Part model, mm, in its own coordinate system. Face numbers are marked on the shaded views. Coordinates: 2 decimals unless noted, no trailing zeros. Loops run counter-clockwise (first coordinate to the right, second up) from the corner with the lowest first, then second, coordinate; pieces in that order, holes last. Notation, with made-up numbers: (18, -25.75) - (71, -25.75) arc R29 ccw to (71, -2.75) - close; hole circle Ø7 at (28.5, 76.5). An arc over 180 degrees is marked (long way). Use a Markdown table: item, result. Add a question column.
1. Wall check: probe 1 along X at (y, z) = (99.5, 0); probe 2 along X at (y, z) = (-85.5, -11); probe 3 along Z at (x, y) = (-12, 92.5). Give the ranges that are in metal, low to high. Write a range as [from, to].
2. Drop flat-ended pins along their axis: pin 1 (5 mm diameter, centred on y = 34.5, z = 10, fed in from +X); pin 2 (2 mm diameter, centred on x = -2, z = -8.5, fed in from -Y); pin 3 (1 mm diameter, centred on x = 12.5, y = 90, fed in from +Z); pin 4 (4 mm diameter, centred on y = -31, z = -18.5, fed in from +X). Give the stop position or say it passes through.
3. Band-saw the part on A-A, the plane x = -10. Give the cut face in (y, z).
4. Pull direction Y, two halves, no side cores. Call the marked faces 1, 2, 3 and 4: pulls with the +Y half, pulls with the -Y half, needs draft (parallel to the pull), parting line crosses it, or undercut.
5. Band-saw the part on C-C, the plane x = 15. Give the cut face in (y, z), plus the area to 3 significant figures.
6. Band-saw the part on B-B, the plane z = 0. Give the cut face in (x, y).
from build123d import *

# Parameters (mm, degrees)
BOSS_EXTRUDE1_DEPTH = 7.5
CHAMFER1_SIZE       = 2.5
SKETCH2_R           = 5
BOSS_EXTRUDE2_DEPTH = 10
BOSS_EXTRUDE3_DEPTH = 5


with BuildPart() as part:
    # Sketch1 → Boss-Extrude1 (new, symmetric)
    with BuildSketch(Plane.YZ):
        with BuildLine():
            ThreePointArc((-81.871756055, 19.753837344), (-104.803696773, 2.795280684), (-87.461525308, -19.847944306))
            ThreePointArc((-87.461525308, -19.847944306), (0.380210023, -22.09713345), (86.984359422, -7.232725467))
            ThreePointArc((86.984359422, -7.232725467), (92.427584063, 1.039709088), (84.922137279, 7.499595816))
            ThreePointArc((84.922137279, 7.499595816), (1.268561005, 10.133701432), (-81.871756055, 19.753837344))
        make_face()
    extrude(amount=BOSS_EXTRUDE1_DEPTH, both=True)

    # Chamfer1
    chamfer1_edges = [part.edges().sort_by_distance(p)[0] for p in [
        (-7.5, 0.380210023, -22.09713345),
        (-7.5, -104.803696773, 2.795280684),
        (-7.5, 1.268561005, 10.133701432),
        (7.5, 0.380210023, -22.09713345),
        (7.5, -104.803696773, 2.795280684),
        (7.5, 1.268561005, 10.133701432),
    ]]
    chamfer(chamfer1_edges, length=CHAMFER1_SIZE)

    # Sketch2 → Boss-Extrude2 (add)
    with BuildSketch(Plane(origin=(-7.5, 0, 0), x_dir=(0, -1, 0), z_dir=(-1, 0, 0))):
        with Locations(Location((85, 0, 0), (0, 0, 270))):
            Circle(SKETCH2_R)
    extrude(amount=BOSS_EXTRUDE2_DEPTH)

    # Sketch4 → Boss-Extrude3 (add, symmetric)
    with BuildSketch(Plane(origin=(0, 0, 0), x_dir=(0, 1, 0), z_dir=(0, 0, 1))):
        with BuildLine():
            ThreePointArc((86.984359422, 0), (95.845428844, -15.310516356), (113.386137378, -17.602678336))
            ThreePointArc((113.386137378, -17.602678336), (115.102678336, -14.113862622), (111.613862622, -12.397321664))
            ThreePointArc((111.613862622, -12.397321664), (99.049040037, -10.836148037), (92.5, 0))
            ThreePointArc((92.5, 0), (99.049040037, 10.836148037), (111.613862622, 12.397321664))
            ThreePointArc((111.613862622, 12.397321664), (115.102678336, 14.113862622), (113.386137378, 17.602678336))
            ThreePointArc((113.386137378, 17.602678336), (95.845428844, 15.310516356), (86.984359422, 0))
        make_face()
    extrude(amount=BOSS_EXTRUDE3_DEPTH, both=True)


solid = part.part
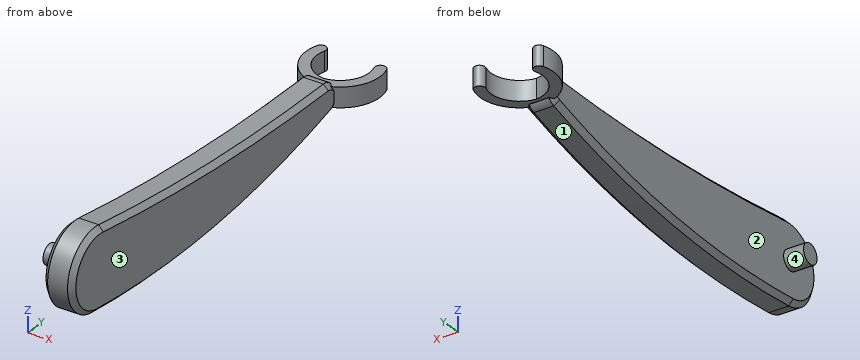
Geometry check:
| question | item | result |
|---|---|---|
| 1 | probe 1 | x = [-17.23, -11.12], [11.12, 17.23] |
| 1 | probe 2 | x = [-7.5, 7.5] |
| 1 | probe 3 | z = [-5, 5] |
| 2 | pin 1 | stops at x = 5.75 |
| 2 | pin 2 | stops at y = -103.54 |
| 2 | pin 3 | passes through |
| 2 | pin 4 | stops at x = 7.5 |
| 3 | outline | circle Ø10 at (-85, 0); (90.46, -5) - (97.89, -5) - (97.89, 5) - (90.46, 5) - close |
| 4 | face 1 | parting line crosses it |
| 4 | face 2 | undercut |
| 4 | face 3 | needs draft |
| 4 | face 4 | undercut |
| 5 | outline | (95.39, -5) - (115.25, -5) - (115.25, 5) - (95.39, 5) - close |
| 5 | area | 199 mm^2 |
| 6 | outline | (-17.6, 113.39) arc R20 ccw to (-7.5, 88.99) - (-7.5, -80) - (-17.5, -80) - (-17.5, -90) - (-7.5, -90) - (-7.5, -102.5) - (-5, -105) - (5, -105) - (7.5, -102.5) - (7.5, 88.99) arc R20 ccw to (17.6, 113.39) arc R2.75 ccw to (12.4, 111.61) arc R14.5 cw to (0, 92.5) arc R14.5 cw to (-12.4, 111.61) arc R2.75 ccw to start |
